The figure shows three views and two pictorial views of one solid part (mm, origin at its lowest corner). Answer the questions. Coordinates: 2 decimals unless noted, no trailing zeros. Loops run counter-clockwise (first coordinate to the right, second up) from the corner with the lowest first, then second, coordinate; pieces in that order, holes last. Notation, with made-up numbers: (-39.75, 66.5) -> (-26.75, 66.5) arc R17 ccw to (-26.75, 86.5) -> close; hole circle Ø9 at (80.25, -10). An arc over 180 degrees is marked (long way). Answer in a Markdown table with one row per item.
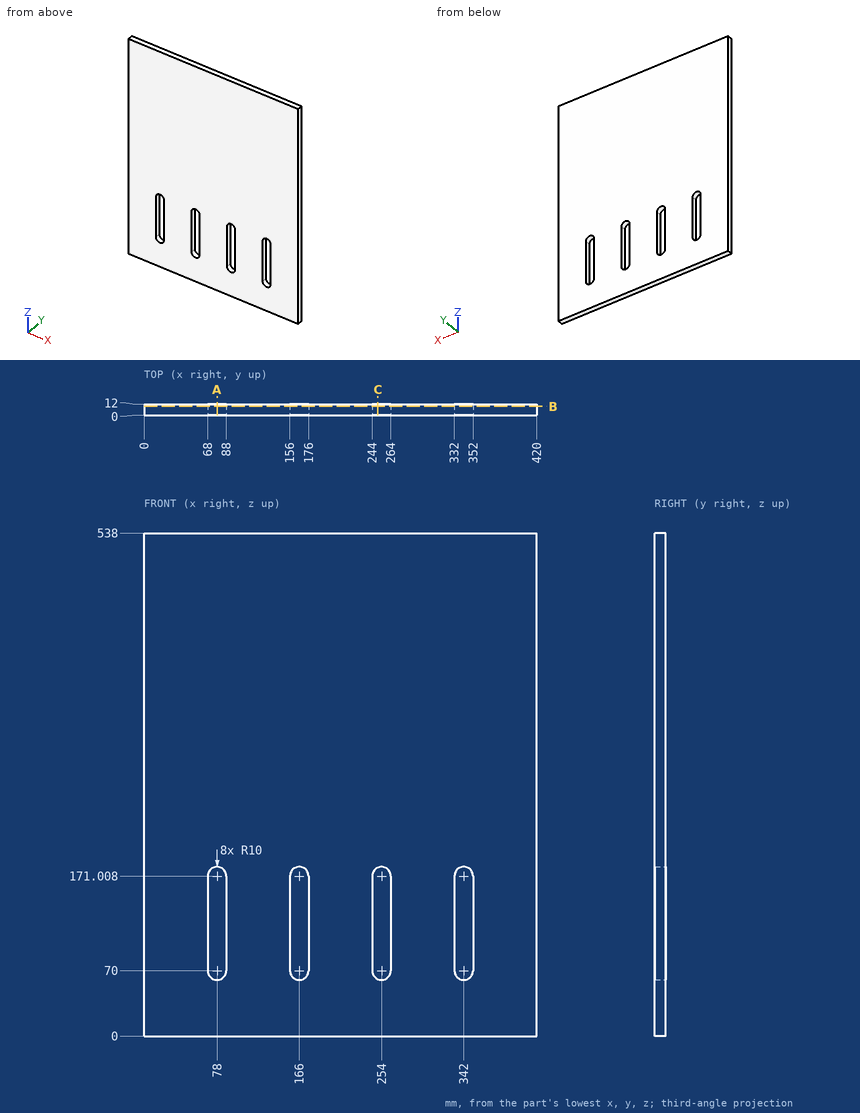
Item 1: Find the intervals of material crossed by probe 1 along X at (y, z) = (7.5, 150.5); probe 2 along X at (y, z) = (10.25, 67.5), in increasing order.
Findings below:
| item | result |
|---|---|
| probe 1 | x = 0 to 68, 88 to 156, 176 to 244, 264 to 332, 352 to 420 |
| probe 2 | x = 0 to 68.32, 87.68 to 156.32, 175.68 to 244.32, 263.68 to 332.32, 351.68 to 420 |
Item 2: A flat-ended cylindrical pin translates along its axis: pin 1 Ø1 at (x, y) = (367, 2.5) entering from -Z. Find the tip coordinate at first contact, or state that the pin passes through.
Findings below:
| item | result |
|---|---|
| pin 1 | stops at z = 0 |
Item 3: A cutting plane is placed at B-B, the plane y = 9.5. Determine the outline of the cut face in (x, z).
Findings below:
| item | result |
|---|---|
| outline | (0, 0) -> (420, 0) -> (420, 538) -> (0, 538) -> close; hole (68, 70) arc R10 ccw to (88, 70) -> (88, 171.01) arc R10 ccw to (68, 171.01) -> close; hole (156, 70) arc R10 ccw to (176, 70) -> (176, 171.01) arc R10 ccw to (156, 171.01) -> close; hole (244, 70) arc R10 ccw to (264, 70) -> (264, 171.01) arc R10 ccw to (244, 171.01) -> close; hole (332, 70) arc R10 ccw to (352, 70) -> (352, 171.01) arc R10 ccw to (332, 171.01) -> close |
Item 4: A cutting plane is placed at A-A, the plane x = 78. Determine the outline of the cut face in (y, z).
Findings below:
| item | result |
|---|---|
| outline | (0, 0) -> (12, 0) -> (12, 60) -> (0, 60) -> close; (0, 181.01) -> (12, 181.01) -> (12, 538) -> (0, 538) -> close |
Item 5: A cutting plane is placed at C-C, the plane x = 250. Determine the outline of the cut face in (y, z) (1 decimal), plus the area to 3 significant figures.
Findings below:
| item | result |
|---|---|
| outline | (0, 0) -> (12, 0) -> (12, 60.8) -> (0, 60.8) -> close; (0, 180.2) -> (12, 180.2) -> (12, 538) -> (0, 538) -> close |
| area | 5,020 mm2 |
